from build123d import *

# Parameters (mm, degrees)
BOSS_EXTRUDE1_DEPTH     = 7
SKETCH2_R               = 1.5
CUT_EXTRUDE1_DEPTH      = 10
MIRROR2_COPY_1_SKETCH_R = 1.5
MIRROR2_COPY_1_DEPTH    = 10
CUT_EXTRUDE4_START      = -8
SKETCH5_R               = 2.5
CUT_EXTRUDE4_DEPTH      = 9
MIRROR6_START           = -8
MIRROR6_COPY_1_SKETCH_R = 2.5
MIRROR6_COPY_1_DEPTH    = 9
CUT_EXTRUDE5_START      = -8
SKETCH6_R               = 2.5
CUT_EXTRUDE5_DEPTH      = 9
MIRROR9_START           = -8
MIRROR9_COPY_1_SKETCH_R = 2.5
MIRROR9_COPY_1_DEPTH    = 9


with BuildPart() as part:
    # Sketch1 → Boss-Extrude1 (new body)
    with BuildSketch(Plane.XY):
        Polygon((-30.22420519, 75.913209403), (30.22420519, 75.913209403), (30.22420519, 88.519824063), (73.519824063, 88.519824063), (73.519824063, 45.22420519), (60.913209403, 45.22420519), (60.913209403, -45.22420519), (73.519824063, -45.22420519), (73.519824063, -88.519824063), (30.22420519, -88.519824063), (30.22420519, -75.913209403), (-30.22420519, -75.913209403), (-30.22420519, -88.519824063), (-73.519824063, -88.519824063), (-73.519824063, -45.22420519), (-60.913209403, -45.22420519), (-60.913209403, 45.22420519), (-73.519824063, 45.22420519), (-73.519824063, 88.519824063), (-30.22420519, 88.519824063), align=None)
        Polygon((-28, 48), (28, 48), (28, 43), (33, 43), (33, -43), (28, -43), (28, -48), (-28, -48), (-28, -43), (-33, -43), (-33, 43), (-28, 43), align=None, mode=Mode.SUBTRACT)
    extrude(amount=BOSS_EXTRUDE1_DEPTH)

    # Sketch2 → Cut-Extrude1 (cut)
    with BuildSketch(Plane.XY.offset(7)):
        with Locations((30.5, -45.5)):
            Circle(SKETCH2_R)
    cut_extrude1 = extrude(amount=-CUT_EXTRUDE1_DEPTH, mode=Mode.SUBTRACT)

    # Mirror1: Cut-Extrude1 across plane
    add(cut_extrude1.mirror(Plane(origin=(0, 0, 0), x_dir=(0, 0, 1), z_dir=(1, 0, 0))), mode=Mode.SUBTRACT)

    # Mirror2: Cut-Extrude1 across plane
    add(cut_extrude1.mirror(Plane.ZX), mode=Mode.SUBTRACT)

    # Mirror2 copy 1 sketch → Mirror2 copy 1 (cut)
    with BuildSketch(Plane(origin=(0, 0, 7), x_dir=(-1, 0, 0), z_dir=(0, 0, 1))):
        with Locations((30.5, -45.5)):
            Circle(MIRROR2_COPY_1_SKETCH_R)
    extrude(amount=-MIRROR2_COPY_1_DEPTH, mode=Mode.SUBTRACT)

    # Sketch5 → Cut-Extrude4 (cut)
    with BuildSketch(Plane.XY.offset(7).offset(CUT_EXTRUDE4_START)):
        with Locations((-45, 75)):
            Circle(SKETCH5_R)
    cut_extrude4 = extrude(amount=CUT_EXTRUDE4_DEPTH, mode=Mode.SUBTRACT)

    # Mirror5: Cut-Extrude4 across plane
    add(cut_extrude4.mirror(Plane.ZX), mode=Mode.SUBTRACT)

    # Mirror6: Cut-Extrude4 across plane
    add(cut_extrude4.mirror(Plane(origin=(0, 0, 0), x_dir=(0, 0, 1), z_dir=(1, 0, 0))), mode=Mode.SUBTRACT)

    # Mirror6 copy 1 sketch → Mirror6 copy 1 (cut)
    with BuildSketch(Plane(origin=(0, 0, 7), x_dir=(-1, 0, 0), z_dir=(0, 0, 1)).offset(MIRROR6_START)):
        with Locations((-45, 75)):
            Circle(MIRROR6_COPY_1_SKETCH_R)
    extrude(amount=MIRROR6_COPY_1_DEPTH, mode=Mode.SUBTRACT)

    # Sketch6 → Cut-Extrude5 (cut)
    with BuildSketch(Plane(origin=(0, 0, 0), x_dir=(-1, 0, 0), z_dir=(0, 0, -1)).offset(CUT_EXTRUDE5_START)):
        with Locations((63.519824063, 58.519824063)):
            Circle(SKETCH6_R)
    cut_extrude5 = extrude(amount=CUT_EXTRUDE5_DEPTH, mode=Mode.SUBTRACT)

    # Mirror8: Cut-Extrude5 across plane
    add(cut_extrude5.mirror(Plane(origin=(0, 0, 0), x_dir=(0, 0, 1), z_dir=(1, 0, 0))), mode=Mode.SUBTRACT)

    # Mirror9: Cut-Extrude5 across plane
    add(cut_extrude5.mirror(Plane.ZX), mode=Mode.SUBTRACT)

    # Mirror9 copy 1 sketch → Mirror9 copy 1 (cut)
    with BuildSketch(Plane(origin=(0, 0, 0), x_dir=(1, 0, 0), z_dir=(0, 0, -1)).offset(MIRROR9_START)):
        with Locations((63.519824063, 58.519824063)):
            Circle(MIRROR9_COPY_1_SKETCH_R)
    extrude(amount=MIRROR9_COPY_1_DEPTH, mode=Mode.SUBTRACT)


solid = part.part
Here's how the part is built. I have some questions about the finished solid (model axes, mm). A direction names the side the tool comes from. Coordinates: 2 decimals unless noted, no trailing zeros. Loops run counter-clockwise (first coordinate to the right, second up) from the corner with the lowest first, then second, coordinate; pieces in that order, holes last. Notation, with made-up numbers: (89, 67) -> (96, 67) arc R27 cw to (96, 100) -> close; hole circle Ø7 at (43.25, -0.75). An arc over 180 degrees is marked (long way). Use one line per item in the form item = value. Start each with the question number.
(1) If we section it at A-A (y = -40): Please give me the cut outline in (x, z).
(2) If we section it at D-D (z = 3.5): Give the number of separate pieces and of enclosed holes in the cut face, then the cut area to 3 significant figures.
(3) On a 3-axis mill with a long thin cutter (end or side, diameter ignored), from which of +Z, -Z, +X, -X, +Y, -Y can I reach the whole of each face in a straight line? I mean faces 1 (the face through (33, 1, 3)), 2 (the face through (52, -88.52, 3)), 3 (the face through (-52, 88.52, 3)), 4 (the face through (67, -45.224, 3)), 5 (the face through (-67, 45.224, 3)). Say none if no direction works.
(4) If we section it at C-C (x = 45): Please give me the cut outline in (y, z), then the cut area to 3 significant figures.
(5) Please list where these lines run through material, in increasing order: line 1 along X through (y, z) = (45.5, 5.5); line 2 along Y through (x, z) = (-45, 2.75); line 3 along X through (y, z) = (-4.5, 0.5).
(6) We'd pull the mould along Y, two halves only. Please class faces 6 (the face through (31, -43, 3)), 7 (the face through (34, 1, 7)), 8 (the face through (0, -75.913, 3)): pulls with the +Y half, pulls with the -Y half, needs draft (parallel to the pull), parting line crosses it, or undercut.
(7) If we section it at B-B (x = -11): Please give me the cut outline in (y, z).
(8) Will these pins go through, and if not, where does the flat tip stop? pin 1 (3 mm diameter, centred on x = -11.5, z = 4, fed in from -Y); pin 2 (3.5 mm diameter, centred on x = 11, z = 5, fed in from +Y); pin 3 (1 mm diameter, centred on y = -29, z = 5, fed in from -X); pin 4 (3 mm diameter, centred on x = -45, y = 75, fed in from +Z).
Verdict:
q1.outline = (-60.91, 0) -> (-33, 0) -> (-33, 7) -> (-60.91, 7) -> close; (33, 0) -> (60.91, 0) -> (60.91, 7) -> (33, 7) -> close
q2.separate_pieces = 1
q2.enclosed_holes = 13
q2.area = 15,800 mm²
q3.face_1 = +Z, -Z
q3.face_2 = +Z, -Z, +X, -X, -Y
q3.face_3 = +Z, -Z, +X, -X, +Y
q3.face_4 = +Z, -Z, +X
q3.face_5 = +Z, -Z, -X
q4.outline = (-88.52, 0) -> (-77.5, 0) -> (-77.5, 7) -> (-88.52, 7) -> close; (-72.5, 0) -> (72.5, 0) -> (72.5, 7) -> (-72.5, 7) -> close; (77.5, 0) -> (88.52, 0) -> (88.52, 7) -> (77.5, 7) -> close
q4.area = 1,170 mm²
q5.line_1 = -73.52 to -32, -29 to -28, 28 to 29, 32 to 73.52
q5.line_2 = -88.52 to -77.5, -72.5 to 72.5, 77.5 to 88.52
q5.line_3 = -60.91 to -33, 33 to 60.91
q6.face_6 = undercut
q6.face_7 = needs draft
q6.face_8 = pulls with the -Y half
q7.outline = (-75.91, 0) -> (-48, 0) -> (-48, 7) -> (-75.91, 7) -> close; (48, 0) -> (75.91, 0) -> (75.91, 7) -> (48, 7) -> close
q8.pin_1 = -75.91
q8.pin_2 = 75.91
q8.pin_3 = -60.91
q8.pin_4 = through
